Study the drawing (mm; zero at the part's minimum x, y, z) and answer. A direction names the side the tool comes from. Coordinates: 2 decimals unless noted, no trailing zeros. Order: outer loops, then holes, each group sorted by start corner. A loop starts at its lowest first (then second) coordinate and runs counter-clockwise, first axis right, second up. Notation, with made-up numbers: M -31,84 L -22,84 A16 ccw -22,98 Z; hole C 43.25,43 d2. An arc over 180 degrees is marked long. Put each result on its own line as item: value.
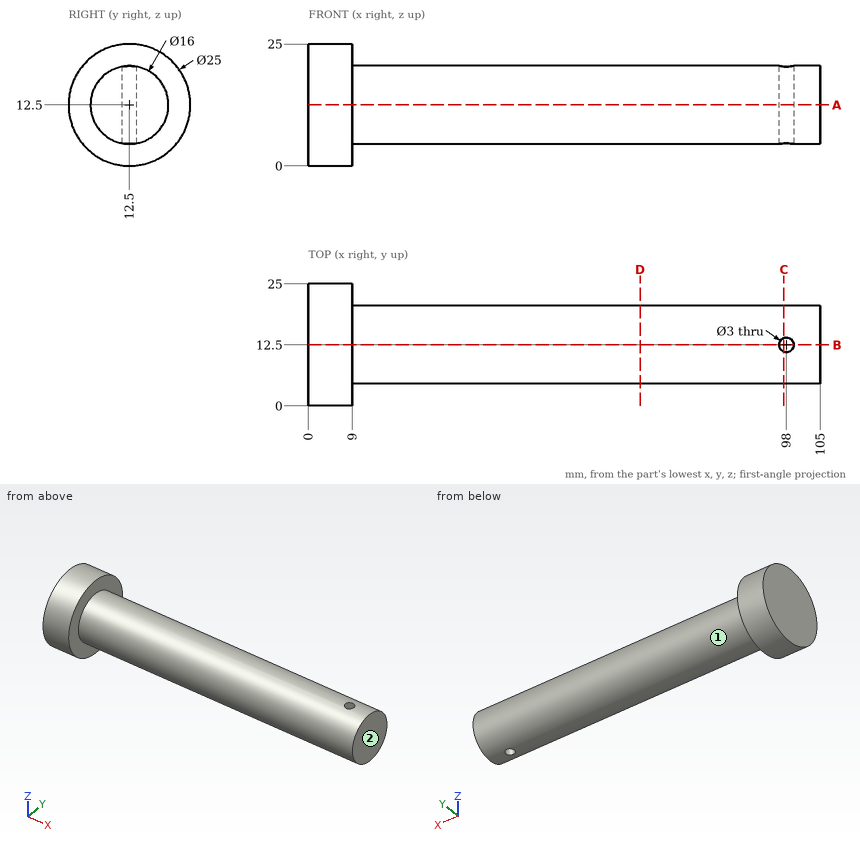
Q1. Find section C-C on x = 97.5. Write down the section's boundary in (y, z), plus the area to 3 significant figures.
Answers below:
outline: M 11.09,4.63 L 11.09,20.37 A8 ccw Z; M 13.91,4.63 A8 ccw 13.91,20.37 Z
area: 156 mm^2
Q2. Given pin 1 (8 mm diameter, centred on x = 81.5, y = 12, fed in from +Z); pin 2 (4 mm diameter, centred on x = 77.5, y = 9, fed in from -Z); pin 3 (5 mm diameter, centred on x = 88.5, z = 14.5, fed in from -Y); pin 4 (1.8 mm diameter, centred on x = 98, y = 12.5, fed in from +Z), each flat-ended and moving along its own axis, determine where each tip first touches the part or whether it passes through.
Answers below:
pin 1: stops at z = 20.5
pin 2: stops at z = 4.64
pin 3: stops at y = 4.5
pin 4: passes through
Q3. Find section B-B on y = 12.5. Write down the section's boundary in (x, z).
Answers below:
outline: M 0,0 L 9,0 L 9,4.5 L 96.5,4.5 L 96.5,20.5 L 9,20.5 L 9,25 L 0,25 Z; M 99.5,4.5 L 105,4.5 L 105,20.5 L 99.5,20.5 Z
Q4. Find section D-D on x = 68. Write down the section's boundary in (y, z).
Answers below:
outline: C 12.5,12.5 d16
Q5. A tool of negligible diameter and unlimited length cuts with its end or side. For the marked faces 1 and 2, from which of +Z, -Z, +X, -X, +Y, -Y can it reach the whole face along a straight path? Write none if from no direction.
Answers below:
face 1: +X
face 2: +Z, -Z, +X, +Y, -Y
Q6. Consider line 1 along X through (y, z) = (12.5, 10.75); line 2 along Y through (x, z) = (98, 12.75); line 3 along Z through (x, y) = (36, 12). Determine where each line is inside the solid, lowest interval first.
Answers below:
line 1: x = 0 to 96.5, 99.5 to 105
line 2: y = 4.5 to 11, 14 to 20.5
line 3: z = 4.52 to 20.48
Q7. Find section A-A on z = 12.5. Write down the section's boundary in (x, y), plus the area to 3 significant figures.
Answers below:
outline: M 0,0 L 9,0 L 9,4.5 L 105,4.5 L 105,20.5 L 9,20.5 L 9,25 L 0,25 Z; hole C 98,12.5 d3
area: 1,750 mm^2
